The listing builds one solid part. Answer for the finished solid, in the listing's coordinates (mm). Face numbers are marked on the shaded views. Round coordinates to 2 decimals unless told otherwise and drop trailing zeros. Loops run counter-clockwise (first coordinate to the right, second up) from the corner with the lowest first, then second, coordinate; pieces in that order, holes last. Notation, with made-up numbers: (-36, 9) -> (-21, 9) arc R36 cw to (-21, 46) -> close; hole circle Ø5 at (-40, 41). An arc over 180 degrees is marked (long way). Answer in a Markdown table with one row per item. Add a question column.
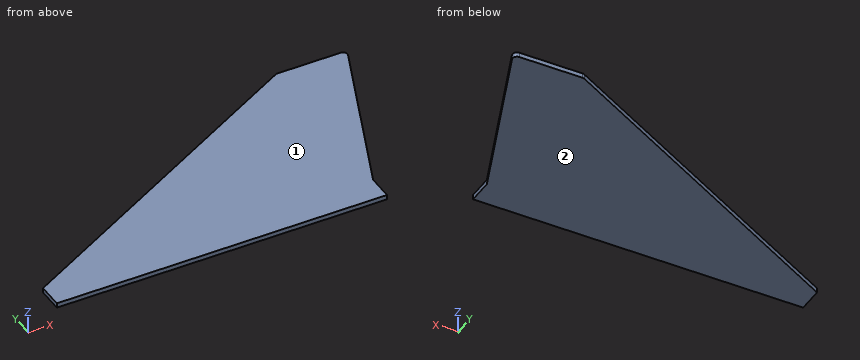
```python
from build123d import *

# Parameters (mm, degrees)
FIN_BODY_DEPTH = 5.08
FIN_FILLETS_R  = 4.7625


with BuildPart() as part:
    # Fin Profile → Fin Body (new body)
    with BuildSketch(Plane.XY):
        Polygon((355.6, -27.2542), (0, -27.2542), (0, 0), (355.6, 190.5), (431.8, 190.5), (355.6, 0), align=None)
    extrude(amount=FIN_BODY_DEPTH)

    # Fin Fillets
    fin_fillets_edges = [part.edges().sort_by_distance(p)[0] for p in [
        (431.8, 190.5, 2.54),
        (355.6, 190.5, 2.54),
    ]]
    fillet(fin_fillets_edges, radius=FIN_FILLETS_R)


solid = part.part
```
Item 1: Section C-C, the plane x = 389 is taken. Write down the section's boundary in (y, z).
Item 2: Section B-B, the plane y = 94.5 is taken. Write down the section's boundary in (x, z).
Item 3: Flat-ended cylindrical pins translate along their axes: P1, Ø1.5, axis at y = 117, z = 4, coming from the -X side; P2, Ø2, axis at y = 65.5, z = 1, coming from the -X side; P3, Ø1.5, axis at x = 136.5, z = 0.5, coming from the +Y side. Find the tip coordinate at first contact, or state that the pin passes through.
Item 4: The mould has two halves that part along Z. Classify the marked faces 1 and 2: +Z half, -Z half, draft (parallel to the pull), parting line (faces both ways), or undercut.
Item 5: Consider L1, parallel to X at y = 71.5, z = 2.45; L2, parallel to Y at x = 213, z = 1; L3, parallel to X at y = 51, z = 0.85. Determine where each line is inside the solid, lowest interval first. Write a range as from..to.
Item 6: Section A-A, the plane z = 3.8 is taken. Write down the section's boundary in (x, y) (1 decimal).
Here are the results:
| question | item | result |
|---|---|---|
| 1 | outline | (83.5, 0) -> (190.5, 0) -> (190.5, 5.08) -> (83.5, 5.08) -> close |
| 2 | outline | (176.4, 0) -> (393.4, 0) -> (393.4, 5.08) -> (176.4, 5.08) -> close |
| 3 | P1 | stops at x = 217 |
| 3 | P2 | stops at x = 120.4 |
| 3 | P3 | stops at y = 73.53 |
| 4 | face 1 | +Z half |
| 4 | face 2 | -Z half |
| 5 | L1 | x = 133.47..384.2 |
| 5 | L2 | y = -27.25..114.11 |
| 5 | L3 | x = 95.2..376 |
| 6 | outline | (0, -27.3) -> (355.6, -27.3) -> (355.6, 0) -> (429.2, 184) arc R4.8 ccw to (424.8, 190.5) -> (356.8, 190.5) arc R4.8 ccw to (354.5, 189.9) -> (0, 0) -> close |
